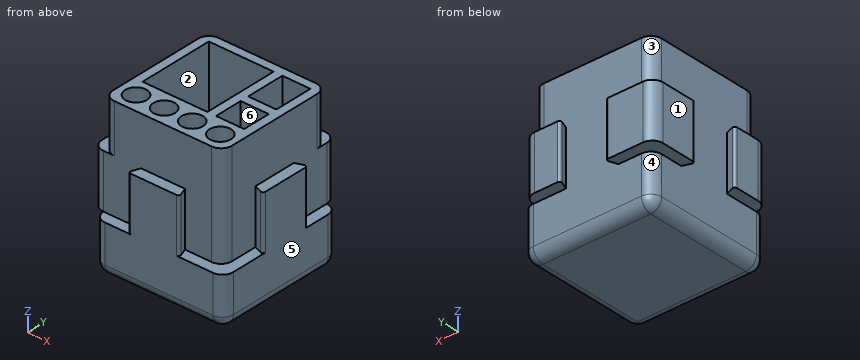
```python
from build123d import *

# Parameters (mm, degrees)
F1_DEPTH = 35
F0_W     = 5.1
F0_H     = 5.1
F2_DEPTH = 12.5
F4_DEPTH = 22.5
F5_R     = 5
F6_R     = 1
F7_W     = 30
F7_H     = 35
F7_R     = 5
F7_W_2   = 13
F7_H_2   = 18
F7_H_3   = 13
F8_DEPTH = 65
F9_DEPTH = 25


with BuildPart() as f1:
    # F0 (on Top) → F1 (new body, symmetric)
    with BuildSketch(Plane.XY):
        Polygon((-11.9, 27.5), (-27.5, 27.5), (-27.5, 12.3), (-27.5, -11.9), (-27.5, -27.5), (-10.1801488287, -27.5), (10.1801488287, -27.5), (27.5, -27.5), (27.5, -10.1801488287), (27.5, 10.1801488287), (27.5, 27.5), (12.3, 27.5), align=None)
    extrude(amount=F1_DEPTH, both=True)

    # F0 (on Top) → F2 (join, symmetric)
    with BuildSketch(Plane.XY):
        Polygon((-27.5, 12.3), (-27.5, 27.5), (-32.6, 27.5), (-32.6, 10.4437518052), align=None)
        Polygon((-27.5, -27.5), (-27.5, -11.9), (-32.6, -10.0437518052), (-32.6, -27.5), align=None)
        Polygon((-27.5, 32.6), (-27.5, 27.5), (-11.9, 27.5), (-10.0437518052, 32.6), align=None)
        Polygon((10.4437518052, 32.6), (12.3, 27.5), (27.5, 27.5), (27.5, 32.6), align=None)
        Polygon((10.1801488287, -27.5), (-10.1801488287, -27.5), (-12, -32.5), (12, -32.5), align=None)
        Polygon((32.5, 12), (27.5, 10.1801488287), (27.5, -10.1801488287), (32.5, -12), align=None)
        with Locations((-30.05, 30.05)):
            Rectangle(F0_W, F0_H)
    extrude(amount=F2_DEPTH, both=True)

    # F3 (on face) → F4 (join, through all)
    with BuildSketch(Plane(origin=(0, 0, -35), x_dir=(1, 0, 0), z_dir=(0, 0, -1))):
        Polygon((-27.5, 32.5), (-27.5, 27.5), (27.5, 27.5), (27.5, -27.5), (32.5, -27.5), (32.5, 32.5), align=None)
    extrude(amount=-F4_DEPTH)

    # F5
    f5_edges = [f1.edges().sort_by_distance(p)[0] for p in [
        (-32.6, 32.6, 0),
        (-27.5, 27.5, 23.75),
        (-27.5, 27.5, -23.75),
        (-32.6, -27.5, 0),
        (-27.5, -32.5, -23.75),
        (32.5, -32.5, -23.75),
        (27.5, -27.5, 11.25),
        (32.5, 27.5, -23.75),
        (27.5, 32.6, 0),
        (27.5, 27.5, 23.75),
        (32.5, -2.5, -35),
        (2.5, -32.5, -35),
        (-27.5, -2.5, -35),
        (2.5, 27.5, -35),
        (-27.5, -27.5, 23.75),
    ]]
    fillet(f5_edges, radius=F5_R)

    # F6
    f6_edges = [f1.edges().sort_by_distance(p)[0] for p in [
        (12, -32.5, 0),
        (-12, -32.5, 0),
        (32.5, -12, 0),
        (32.5, 12, 0),
        (10.443752, 32.6, 0),
        (-10.043752, 32.6, 0),
        (-32.6, 10.443752, 0),
        (-32.6, -10.043752, 0),
    ]]
    fillet(f6_edges, radius=F6_R)

    # F7 (on face) → F8 (cut)
    with BuildSketch(Plane.XY.offset(35)):
        with Locations((-8.5, 6)):
            Rectangle(F7_W, F7_H)
        with Locations((-6.5, -19.5)):
            Circle(F7_R)
        with Locations((6.5, -19.5)):
            Circle(F7_R)
        with Locations((17, 14.5)):
            Rectangle(F7_W_2, F7_H_2)
        with Locations((17, -5)):
            Rectangle(F7_W_2, F7_H_3)
        with Locations((19.5, -19.5)):
            Circle(F7_R)
    extrude(amount=-F8_DEPTH, mode=Mode.SUBTRACT)

    # F7 (on face) → F9 (cut)
    with BuildSketch(Plane.XY.offset(35)):
        with Locations((-19.5, -19.5)):
            Circle(F7_R)
    extrude(amount=-F9_DEPTH, mode=Mode.SUBTRACT)


solid = f1.part
```
Check sheet for the modelled part. Datum: model origin and axes. Units: mm. Face numbers are marked on the shaded views. A direction names the side the tool comes from. Give positions to 0.01 mm unless a question says otherwise; leave off trailing zeros. Loops run counter-clockwise (first coordinate to the right, second up) from the corner with the lowest first, then second, coordinate; pieces in that order, holes last. Notation, with made-up numbers: M -0.5,49 L 40.5,49 A38 ccw 40.5,88 Z; hole C 80.5,20 d10. An arc over 180 degrees is marked long. Answer as CSV lines item,"result".
Item 1: Depth check by flat-ended pin: pin 1 Ø15 at (x, y) = (-9.5, 9) entering from +Z; pin 2 Ø1.5 at (x, z) = (21, 17.5) entering from -Y; pin 3 Ø2.5 at (x, y) = (-16, -30) entering from +Z. Enter the tip coordinate at first touch or a pass-through.
Reply:
pin 1,"z = -30"
pin 2,"y = -27.5"
pin 3,"z = -12.5"
Item 2: Sectioned sample at A-A, the plane z = -26. Enter the section's corners in (x, y).
Reply:
outline,"M -27.5,-27.5 A5 ccw -22.5,-32.5 L 27.5,-32.5 A5 ccw 32.5,-27.5 L 32.5,22.5 A5 ccw 27.5,27.5 L -22.5,27.5 A5 ccw -27.5,22.5 Z; hole M -23.5,-11.5 L 6.5,-11.5 L 6.5,23.5 L -23.5,23.5 Z; hole C -6.5,-19.5 d10; hole C 6.5,-19.5 d10; hole M 10.5,-11.5 L 23.5,-11.5 L 23.5,1.5 L 10.5,1.5 Z; hole M 10.5,5.5 L 23.5,5.5 L 23.5,23.5 L 10.5,23.5 Z; hole C 19.5,-19.5 d10"
Item 3: Sectioned sample at C-C, the plane x = -19.5. Enter the section's corners in (y, z).
Reply:
outline,"M -32.5,-30 A5 ccw -27.5,-35 L 22.5,-35 A5 ccw 27.5,-30 L 27.5,-12.5 L 32.6,-12.5 L 32.6,12.5 L 27.5,12.5 L 27.5,35 L 23.5,35 L 23.5,-30 L -11.5,-30 L -11.5,35 L -14.5,35 L -14.5,10 L -24.5,10 L -24.5,35 L -27.5,35 L -27.5,-12.5 L -32.5,-12.5 Z"
Item 4: Scan lines: L1, parallel to X at y = 0, z = -29; L2, parallel to X at y = 13, z = -1.5; L3, parallel to Y at x = 19.5, z = -14.5. Record each from-to range of solid material in increasing order.
Reply:
L1,"-27.5 to -23.5, 6.5 to 10.5, 23.5 to 32.5"
L2,"-32.6 to -23.5, 6.5 to 10.5, 23.5 to 27.5"
L3,"-32.5 to -24.5, -14.5 to -11.5, 1.5 to 5.5, 23.5 to 27.5"
Item 5: Set-up check for the marked faces 1, 2 and 3: record each of +Z, -Z, +X, -X, +Y, -Y from which the full face is reachable in a straight line by a thin tool's end or side.
Reply:
face 1,"+Z, -Z, -X, +Y, -Y"
face 2,"+Z"
face 3,"+Z, -X, +Y"
Item 6: Sectioned sample at D-D, the plane z = 11. State how many separate pieces and enclosed holes the cut face has, then the cut area to 3 significant figures.
Reply:
separate pieces,"1"
enclosed holes,"7"
area,"1,810 mm^2"
Item 7: Sectioned sample at B-B, the plane y = 2.5. Enter the section's corners in (x, z).
Reply:
outline,"M -27.5,-30 A5 ccw -22.5,-35 L 27.5,-35 A5 ccw 32.5,-30 L 32.5,12.5 L 27.5,12.5 L 27.5,35 L 6.5,35 L 6.5,-30 L -23.5,-30 L -23.5,35 L -27.5,35 Z"
Item 8: Draft check along Y on the marked faces 4, 5 and 6. Enter one of: pulls with the +Y half, pulls with the -Y half, needs draft (parallel to the pull), parting line crosses it, or undercut.
Reply:
face 4,"pulls with the +Y half"
face 5,"needs draft"
face 6,"undercut"
